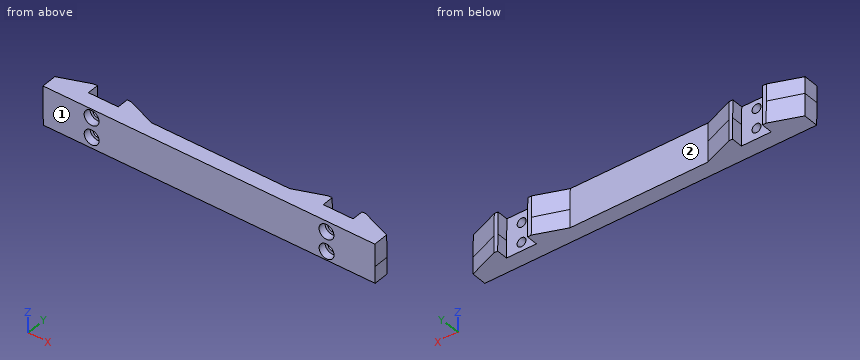
```python
from build123d import *

# Parameters (mm, degrees)
EXTRUDE_1_DEPTH     = 2.5
SKETCH_5_R          = 0.6
CUT_EXTRUDE_1_DEPTH = 19.036421485
CUT_EXTRUDE_START   = -2
SKETCH_5_3_R        = 1
CUT_EXTRUDE_2_DEPTH = 1
REVOLVE_1_ANGLE     = 1
SKETCH_9_R          = 0.6
CUT_EXTRUDE_3_DEPTH = 41.426698916
SKETCH_9_3_R        = 1
CUT_EXTRUDE_4_DEPTH = 1
SKETCH_10_W         = 44.5
SKETCH_10_H         = 2.5
CUT_EXTRUDE_5_DEPTH = 41.528606999
REVOLVE_2_ANGLE     = 1
SKETCH_14_R         = 0.6
CUT_EXTRUDE_6_DEPTH = 41.445950592
SKETCH_14_3_R       = 1
CUT_EXTRUDE_7_DEPTH = 1


with BuildPart() as part:
    # 草图4 → 凸台-拉伸1 (new body)
    with BuildSketch(Plane.XY):
        Polygon((8.5, -1.5), (17.75, -1.5), (17.75, -3.5), (-4.5, -3.5), (-4.5, -1.5), (-0.5, 0), (0, 0), (0, -1.5), (4, -1.5), (4, 0), (4.5, 0), align=None)
    extrude(amount=EXTRUDE_1_DEPTH)

    # 草图5 → 切除-拉伸1 (cut, through all)
    with BuildSketch(Plane(origin=(0, -1.5, 0), x_dir=(1, 0, 0), z_dir=(0, 1, 0))):
        with Locations(Location((2, -1.25, 0), (0, 0, 270))):
            Circle(SKETCH_5_R)
    extrude(amount=-CUT_EXTRUDE_1_DEPTH, mode=Mode.SUBTRACT)

    # 草图5<3> → 切除-拉伸2 (cut)
    with BuildSketch(Plane(origin=(0, -1.5, 0), x_dir=(1, 0, 0), z_dir=(0, 1, 0)).offset(CUT_EXTRUDE_START)):
        with Locations((2, -1.25)):
            Circle(SKETCH_5_3_R)
    extrude(amount=CUT_EXTRUDE_2_DEPTH, mode=Mode.SUBTRACT)

    # 镜向1: part across plane


with BuildPart() as part_1:
    add(part.part)
    add(part.part.mirror(Plane(origin=(17.75, 0, 2.5), x_dir=(0, 0, 1), z_dir=(1, 0, 0))))

    # 草图6 → 旋转1 (revolve)
    with BuildSketch(Plane.XY.offset(2.5)):
        Polygon((0, 0), (-0.5, 0), (-4.5, -1.5), (-4.5, -3.5), (40, -3.5), (40, -1.5), (36, 0), (35.5, 0), (35.5, -1.5), (31.5, -1.5), (31.5, 0), (31, 0), (27, -1.5), (8.5, -1.5), (4.5, 0), (4, 0), (4, -1.5), (0, -1.5), align=None)
    revolve(axis=Axis((-132.25, 94.8535776, 2.5), (0, -1, 0)), revolution_arc=REVOLVE_1_ANGLE)

    # 草图9 → 切除-拉伸3 (cut, through all)
    with BuildSketch(Plane(origin=(0, -1.5, 0), x_dir=(1, 0, 0), z_dir=(0, 1, 0))):
        with Locations(Location((1.994888171, -3.671537391, 0), (0, 0, 180))):
            Circle(SKETCH_9_R)
        with Locations(Location((33.493688748, -3.946423259, 0), (0, 0, 180))):
            Circle(SKETCH_9_R)
    extrude(amount=-CUT_EXTRUDE_3_DEPTH, mode=Mode.SUBTRACT)

    # 草图9<3> → 切除-拉伸4 (cut)
    with BuildSketch(Plane(origin=(0, -1.5, 0), x_dir=(1, 0, 0), z_dir=(0, 1, 0)).offset(CUT_EXTRUDE_START)):
        with Locations((1.994888171, -3.671537391)):
            Circle(SKETCH_9_3_R)
        with Locations((33.493688748, -3.946423259)):
            Circle(SKETCH_9_3_R)
    extrude(amount=CUT_EXTRUDE_4_DEPTH, mode=Mode.SUBTRACT)

    # 草图10 → 切除-拉伸5 (cut, through all)
    with BuildSketch(Plane(origin=(0, 0, 0), x_dir=(1, 0, 0), z_dir=(0, 1, 0))):
        with Locations((17.75, -1.25)):
            Rectangle(SKETCH_10_W, SKETCH_10_H)
    extrude(amount=-CUT_EXTRUDE_5_DEPTH, mode=Mode.SUBTRACT)

    # 草图11 → 旋转2 (revolve)
    with BuildSketch(Plane(origin=(0, 0, 2.5), x_dir=(-1, 0, 0), z_dir=(0, 0, -1))):
        Polygon((0.5, 0), (0, 0), (0, -1.5), (-4, -1.5), (-4, 0), (-4.5, 0), (-8.5, -1.5), (-27, -1.5), (-31, 0), (-31.5, 0), (-31.5, -1.5), (-35.5, -1.5), (-35.5, 0), (-36, 0), (-40, -1.5), (-40, -3.5), (4.5, -3.5), (4.5, -1.5), align=None)
    revolve(axis=Axis((167.75, 63.011743597, 2.5), (0, -1, 0)), revolution_arc=REVOLVE_2_ANGLE)

    # 草图14 → 切除-拉伸6 (cut, through all)
    with BuildSketch(Plane(origin=(0, -1.5, 0), x_dir=(1, 0, 0), z_dir=(0, 1, 0))):
        with Locations(Location((2.006311252, -1.053576741, 0), (0, 0, 180))):
            Circle(SKETCH_14_R)
        with Locations(Location((33.505111829, -1.328462609, 0), (0, 0, 180))):
            Circle(SKETCH_14_R)
    extrude(amount=-CUT_EXTRUDE_6_DEPTH, mode=Mode.SUBTRACT)

    # 草图14<3> → 切除-拉伸7 (cut)
    with BuildSketch(Plane(origin=(0, -1.5, 0), x_dir=(1, 0, 0), z_dir=(0, 1, 0)).offset(CUT_EXTRUDE_START)):
        with Locations((2.006311252, -1.053576741)):
            Circle(SKETCH_14_3_R)
        with Locations((33.505111829, -1.328462609)):
            Circle(SKETCH_14_3_R)
    extrude(amount=CUT_EXTRUDE_7_DEPTH, mode=Mode.SUBTRACT)


solid = part_1.part
```
Work out the finished part from the listing and answer in its coordinate system (mm). Face numbers are marked on the shaded views. A direction names the side the tool comes from. Give positions to 0.01 mm unless a question says otherwise; leave off trailing zeros. Order: outer loops, then holes, each group sorted by start corner. A loop starts at its lowest first (then second) coordinate and runs counter-clockwise, first axis right, second up.
1. For the marked faces 1 and 2, determine the directions among +Z, -Z, +X, -X, +Y, -Y from which every point of the face is accessible in a straight line to the end or side of a thin tool.
Result sheet:
face 1: +Z, -Z, +X, -X, -Y
face 2: +Z, -Z, +Y
2. Straight lines are drawn through the part: L1, parallel to X at y = -3.25, z = 4.5; L2, parallel to X at y = -1.7, z = 3.75; L3, parallel to Z at x = 0.5, y = -3.05. For each, find the intervals that lie inside material, in ascending order.
Result sheet:
L1: x = -4.52 to 1.43, 2.55 to 32.66, 34.33 to 39.99
L2: x = -4.51 to 1.4, 2.59 to 32.93, 34.06 to 40
L3: z = -0.42 to 4.82
3. Section B-B, the plane x = 22 is taken. Determine the outline of the cut face in (y, z).
Result sheet:
outline: (-3.5, -0.04) - (-1.5, -0.04) - (-1.5, 5.19) - (-3.5, 5.19) - close
4. Section A-A, the plane y = -0.5 is taken. Determine the outline of the cut face in (x, z), and give its area (3 significant figures).
Result sheet:
outline: (-1.85, 4.78) arc R130.42 cw to (-1.83, 2.5) arc R169.58 ccw to (-1.81, -0.46) - (0.03, -0.43) arc R167.75 cw to (0, 2.5) arc R132.25 ccw to (-0.02, 4.81) - close; (3.98, 4.88) arc R136.25 cw to (4, 2.5) arc R163.75 ccw to (4.02, -0.36) - (5.86, -0.33) arc R161.92 cw to (5.83, 2.5) arc R138.08 ccw to (5.81, 4.91) - close; (29.64, 5.33) arc R161.92 cw to (29.67, 2.5) arc R138.08 ccw to (29.69, 0.09) - (31.52, 0.12) arc R136.25 cw to (31.5, 2.5) arc R163.75 ccw to (31.48, 5.36) - close; (35.47, 5.43) arc R167.75 cw to (35.5, 2.5) arc R132.25 ccw to (35.52, 0.19) - (37.35, 0.22) arc R130.42 cw to (37.33, 2.5) arc R169.58 ccw to (37.31, 5.46) - close
area: 38.4 mm2
5. Each of these flat-tipped pins is pushed along its axis until it touches: P1, Ø1.5, axis at y = -2.5, z = 0.5, coming from the -X side; P2, Ø1.6, axis at x = 1.99, z = 3.67, coming from the -Y side; P3, Ø2, axis at y = -1, z = 3, coming from the +X side. Where does it stop, or does it pass through?
Result sheet:
P1: stops at x = -4.5
P2: stops at y = -2.5
P3: stops at x = 40
